Autodesk Inventor part; units mm, degrees
ref_plane "YZ Plane" through (0, 0, 0) normal (1, 0, 0) x (0, 1, 0)
ref_plane "XZ Plane" through (0, 0, 0) normal (0, 1, 0) x (-1, 0, 0)
ref_plane "XY Plane" through (0, 0, 0) normal (0, 0, 1) x (1, 0, 0)
sketch "Sketch1" plane through (0, 0, 0) normal (0, 1, 0) x (-1, 0, 0)
  line L0 (-10, 109.5) -> (10, 109.5)
  line L1 (10, 109.5) -> (10, -109.5)
  line L2 (10, -109.5) -> (-10, -109.5)
  line L3 (-10, -109.5) -> (-10, 109.5)
  line L4 (-10, 109.5) -> (10, -109.5) construction
  line L5 (10, 109.5) -> (-10, -109.5) construction
  point P0 (0, 0)
  dimension "d0" = 20
  dimension "d1" = 219
extrude "Extrusion1" add sketch "Sketch1" along normal blind 5
chamfer "Chamfer1" distance 3 angle 45 1 edges at (10, 0, 0)
sketch "Sketch3" plane through (-10, 5, 109.5) normal (0, 0, 1) x (1, 0, 0)
  line L0 (20, -2) -> (17, -5)
  line L1 (20, -2) -> (20, 0)
  line L2 (0, 0) -> (20, 0)
  line L3 (0, -5) -> (0, 0)
  line L4 (0, -5) -> (17, -5)
  line L5 (3, -4) -> (8, -4)
  line L6 (8, -4) -> (8, -1)
  line L7 (8, -1) -> (3, -1)
  line L8 (3, -1) -> (3, -4)
  line L9 (3, -4) -> (8, -1) construction
  line L10 (8, -4) -> (3, -1) construction
  point P0 (10, -5)
  point P1 (5.5, -2.5)
  point P2 (0, -2.5)
  dimension "d10" = 5
  dimension "d11" = 3
  dimension "d12" = 3
extrude "Extrusion3" cut sketch "Sketch3" against normal blind 7.1 contours L8 L7 L6 L5
sketch "Sketch4" plane through (10, 5, -109.5) normal (0, 0, -1) x (-1, 0, 0)
  line L0 (12, -1) -> (12, -4)
  line L1 (17, -1) -> (12, -1)
  line L2 (17, -4) -> (17, -1)
  line L3 (12, -4) -> (17, -4)
  line L4 (12.2, -1.2) -> (12.2, -3.8)
  line L5 (12.2, -3.8) -> (16.8, -3.8)
  line L6 (16.8, -3.8) -> (16.8, -1.2)
  line L7 (16.8, -1.2) -> (12.2, -1.2)
  point P0 (10, -5)
  dimension "d15" = 0.2
extrude "Extrusion4" add sketch "Sketch4" along normal blind 7 contours L7 L6 L5 L4
properties part number "SEPARADOR" material "Steel, Mild, Welded"
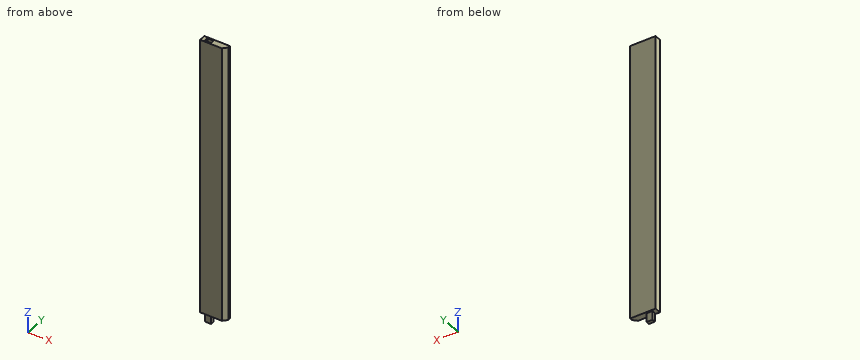
Geometry check sheet. Reference: the model listing, model coordinates, mm. Coordinates: 2 decimals unless noted, no trailing zeros. Order: outer loops, then holes, each group sorted by start corner. A loop starts at its lowest first (then second) coordinate and runs counter-clockwise, first axis right, second up. Notation, with made-up numbers: (21, -6.75) - (66, -6.75) arc R14 cw to (66, 5.25) - close; hole circle Ø1 at (44, 23.5). An arc over 180 degrees is marked (long way). Answer as a JSON object with one key per item and string values. Group by question number.
Item 1: Scan lines: probe 1 along Z at (x, y) = (1.25, 3.15); probe 2 along Z at (x, y) = (-5, 2.8); probe 3 along X at (y, z) = (0.9, 52). Record each from-to range of solid material in increasing order.
Item 2: Depth check by flat-ended pin: pin 1 Ø1.4 at (x, z) = (-5, -114) entering from +Y; pin 2 Ø2 at (y, z) = (2, -112.5) entering from +X; pin 3 Ø0.9 at (x, y) = (-3.5, 2) entering from +Z. Enter the tip coordinate at first touch or a pass-through.
Item 3: Sectioned sample at A-A, the plane z = -102.5. Record the cut outline in (x, y), and give its area (3 significant figures).
Resolved:
{
 "1": {"probe 1": "-109.5 to 109.5", "probe 2": "-116.5 to 102.4", "probe 3": "-10 to 7.9"},
 "2": {"pin 1": "y = 3.8", "pin 2": "x = -2.2", "pin 3": "z = 102.4"},
 "3": {"outline": "(-10, 0) - (7, 0) - (10, 3) - (10, 5) - (-10, 5) - close", "area": "95.5 mm^2"}
}
